Input: part model. Units: mm. Frame: model coordinates. A direction names the side the tool comes from. Give positions to 0.01 mm unless a question says otherwise; leave off trailing zeros. Answer as CSV lines item,"result".
```python
from build123d import *

# Parameters (mm, degrees)
SKETCH6_R               = 1.6
CUT_EXTRUDE3_DEPTH      = 25.4
F_1_4_20_TAPPED_HOLE2_D = 5.1054
SKETCH20_R              = 4
CUT_EXTRUDE4_DEPTH      = 7.81


with BuildPart() as part:
    # Sketch1 → Revolve3 (revolve)
    with BuildSketch(Plane.XY, mode=Mode.PRIVATE) as revolve3_sk:
        with BuildLine():
            Line((12.463542917, 0), (22.464939564, 0))
            Line((22.464939564, 0), (22.464939564, 3))
            ThreePointArc((22.464939564, 3), (12.055156212, 3.701585346), (2.464939564, 7.810545811))
            Line((2.464939564, 7.810545811), (2.464939564, 8.810545811))
            Line((2.464939564, 8.810545811), (-11.305060436, 8.810545811))
            Line((-11.305060436, 8.810545811), (-11.305060436, 7.810545811))
            ThreePointArc((-11.305060436, 7.810545811), (0.993128192, 5.164789847), (12.463542917, 0))
        make_face()
    revolve(revolve3_sk.sketch.rotate(Axis((22.464939564, 0, 0), (0, 1, 0)), 270), axis=Axis((22.464939564, 0, 0), (0, 1, 0)))

    # Sketch6 → Cut-Extrude3 (cut)
    with BuildSketch(Plane(origin=(0, 0, 0), x_dir=(-1, 0, 0), z_dir=(0, -1, 0))):
        with Locations(Location((-2.240445209, -17.721228176, 0), (0, 0, 90))):
            Circle(SKETCH6_R)
        with Locations(Location((-47.924220529, -8.654311802, 0), (0, 0, 90))):
            Circle(SKETCH6_R)
        with Locations(Location((-17.230152955, 26.375539978, 0), (0, 0, 90))):
            Circle(SKETCH6_R)
        with BuildLine():
            Line((-17.074884782, -8.424681994), (-2.715259327, -30.868846833))
            ThreePointArc((-2.715259327, -30.868846833), (-20.776195295, -36.607153906), (-39.28873242, -32.556037354))
            Line((-39.28873242, -32.556037354), (-27.060394573, -8.883116036))
            ThreePointArc((-27.060394573, -8.883116036), (-22.006259237, -9.990874316), (-17.074884782, -8.424681994))
        make_face()
        with BuildLine():
            Line((-32.455682979, -0.461498547), (-58.753919723, -1.676282828))
            Line((-58.753919723, -1.676282828), (-59.072986342, -1.669301437))
            ThreePointArc((-59.072986342, -1.669301437), (-55.012037933, 16.841082029), (-42.247399134, 30.847851619))
            Line((-42.247399134, 30.847851619), (-27.860216814, 8.421339739))
            Line((-27.860216814, 8.421339739), (-27.865844062, 8.417729237))
            ThreePointArc((-27.865844062, 8.417729237), (-31.349526098, 4.592608955), (-32.455682979, -0.461498547))
        make_face()
        with BuildLine():
            Line((-17.869237322, 8.882986874), (-5.772152998, 32.265320109))
            Line((-5.772152998, 32.265320109), (-5.606573626, 32.538149211))
            ThreePointArc((-5.606573626, 32.538149211), (8.393414485, 19.766072993), (14.141313375, 1.708186727))
            Line((14.141313375, 1.708186727), (-12.474206792, 0.46177729))
            Line((-12.474206792, 0.46177729), (-12.474519954, 0.46845588))
            ThreePointArc((-12.474519954, 0.46845588), (-14.045330272, 5.397973163), (-17.869237322, 8.882986874))
        make_face()
    extrude(amount=-CUT_EXTRUDE3_DEPTH, mode=Mode.SUBTRACT)

    # 1/4-20 Tapped Hole2 (through all)
    with Locations(Plane(origin=(0, 0, 0), x_dir=(-1, 0, 0), z_dir=(0, -1, 0))):
        with Locations((-22.464939564, 0)):
            Hole(F_1_4_20_TAPPED_HOLE2_D / 2)

    # Sketch20 → Cut-Extrude4 (cut)
    with BuildSketch(Plane(origin=(0, 0, 0), x_dir=(1, 0, 0), z_dir=(0, 1, 0))):
        with Locations(Location((2.240445209, -17.721228176, 0), (0, 0, 135.127097567))):
            Circle(SKETCH20_R)
        with Locations(Location((17.230152955, 26.375539978, 0), (0, 0, 135.575274994))):
            Circle(SKETCH20_R)
        with Locations(Location((47.924220529, -8.654311802, 0), (0, 0, 136.896542352))):
            Circle(SKETCH20_R)
    extrude(amount=CUT_EXTRUDE4_DEPTH, mode=Mode.SUBTRACT)


solid = part.part
```
Item 1: Reachability of faces 1 (the face through (11.649, 5.69, 16.906)), 2 (the face through (2.306, 6.016, -0.938)), 3 (the face through (44.32, 6.94, 6.92)), 4 (the face through (31.316, 1.778, -4.658)), 5 (the face through (4.636, 8.318, 9.062)) from +Z, -Z, +X, -X, +Y, -Y: full face, straight path, thin tool, end or side. Return the list, or none.
The answers:
face 1,"+Z, +Y, -Y"
face 2,"-Z, +Y, -Y"
face 3,"-Y"
face 4,"+X, +Y, -Y"
face 5,"+Y"
Item 2: Ray query, line 1 (X direction, y = 8.25, z = 10); line 2 (Y direction, x = 25, z = -2.5); line 3 (Y direction, x = 43.5, z = 8). Return the intervals inside material, ascending. Write a range as from..to.
The answers:
line 1,"-9.79..5.14, 39.79..47.06, 48.79..54.72"
line 2,"0..2.84"
line 3,"5.49..8.81"
Item 3: Contact query for flat-ended pins moving along their axis: pin 1 (2.5 mm diameter, centred on x = 3.5, z = 18, fed in from -Y); pin 2 (8 mm diameter, centred on x = 27.5, z = -5, fed in from +Y); pin 3 (5 mm diameter, centred on x = 2.24, z = 17.72, fed in from +Y); pin 4 (4 mm diameter, centred on y = 7.5, z = 16.5, fed in from -X). Output: stop coordinate, or through.
The answers:
pin 1,"y = 7.81"
pin 2,"y = 3.75"
pin 3,"y = 8.81"
pin 4,"x = -8.02"
